Geometry: final body of the model. Coordinates: model frame, mm. A direction names the side the tool comes from. Round coordinates to 2 decimals unless told otherwise and drop trailing zeros. Loops run counter-clockwise (first coordinate to the right, second up) from the corner with the lowest first, then second, coordinate; pieces in that order, holes last. Notation, with made-up numbers: (6, 71) - (54, 71) arc R32 cw to (54, 106) - close; hole circle Ø9 at (56, -12). An arc over 180 degrees is marked (long way). Answer as CSV lines item,"result".
Autodesk Inventor part; units mm, degrees
ref_plane "YZ Plane" through (0, 0, 0) normal (1, 0, 0) x (0, 1, 0)
ref_plane "XZ Plane" through (0, 0, 0) normal (0, 1, 0) x (-1, 0, 0)
ref_plane "XY Plane" through (0, 0, 0) normal (0, 0, 1) x (1, 0, 0)
sketch "Sketch1" plane through (0, 0, 0) normal (1, 0, 0) x (0, 1, 0)
  line L0 (0, 0) -> (44.45, 0)
  line L1 (44.45, 0) -> (44.45, -6.35)
  line L2 (44.45, -6.35) -> (6.35, -6.35)
  line L3 (6.35, -6.35) -> (6.35, -19.05)
  line L4 (6.35, -19.05) -> (0, -19.05)
  line L5 (0, -19.05) -> (0, 0)
  dimension "d0" = 6.35
  dimension "d1" = 44.45
  dimension "d21" = 19.05
extrude "Extrusion1" add sketch "Sketch1" along normal blind 44.45
sketch "Sketch2" plane through (0, 0, 0) normal (0, 0, 1) x (1, 0, 0)
  line L0 (0, 44.45) -> (44.45, 44.45) construction
  line L1 (22.225, 44.45) -> (22.225, 0) construction
  line L2 (0, 0) -> (44.45, 0) construction
  point P0 (22.225, 34.925)
  dimension "d4" = 9.525
hole "Hole1" at (22.225, 34.925, 0) direction (0, 0, -1) diameter 6.7564 end through all
sketch "Sketch4" plane through (0, 6.35, -6.35) normal (0, 1, 0) x (1, 0, 0)
  line L0 (0, 6.35) -> (44.45, 6.35) construction
  line L1 (44.45, -6.35) -> (44.45, 12.7) construction
  line L2 (0, 12.7) -> (44.45, 12.7)
  line L3 (0, 0) -> (0, 12.7)
  point P0 (0, -6.35)
  point P1 (22.225, 6.35)
  point P2 (6.35, 6.35)
  point P3 (38.1, 6.35)
  dimension "d22" = 6.35
  dimension "d23" = 6.35
  dimension "d24" = 6.35
hole "Hole3" at (22.225, 6.35, -12.7) at (6.35, 6.35, -12.7) at (38.1, 6.35, -12.7) direction (0, -1, 0) diameter 5.1054 end through all
properties part number "AngleBracketForEndOfArm"
(1) Section B-B (z = -12.7). Output: boundary loops of the cut face in (x, y).
Findings below:
outline,"(0, 0) - (3.8, 0) - (3.8, 6.35) - (0, 6.35) - close; (8.9, 0) - (19.67, 0) - (19.67, 6.35) - (8.9, 6.35) - close; (24.78, 0) - (35.55, 0) - (35.55, 6.35) - (24.78, 6.35) - close; (40.65, 0) - (44.45, 0) - (44.45, 6.35) - (40.65, 6.35) - close"
(2) Access query for faces 1 (the face through (21.9, 6.35, -15.4)), 2 (the face through (22, 44.45, -3)). Directions: +Z, -Z, +X, -X, +Y, -Y. A direction counts if a zero-diameter tool reaches every point of the face in a straight line with its end or side. Return the directions, or none.
Findings below:
face 1,"-Z, +X, -X, +Y"
face 2,"+Z, -Z, +X, -X, +Y"
(3) Pin query (flat end, axial travel): P1, Ø11.5, axis at x = 19.5, y = 33, coming from the -Z side; P2, Ø1, axis at x = 15, z = -13.5, coming from the +Y side. Return the tip coordinate at first contact, or that it passes through.
Findings below:
P1,"z = -6.35"
P2,"y = 6.35"
(4) Draft query along X for faces 3 (the face through (44.45, 17, -5)), 4 (the face through (22, 22, 0)), 5 (the face through (35.57, 3.13, -13.03)). Return one class per face: pulls with the +X half, pulls with the -X half, needs draft (parallel to the pull), parting line crosses it, or undercut.
Findings below:
face 3,"pulls with the +X half"
face 4,"needs draft"
face 5,"undercut"
(5) Section A-A (x = 38.1). Output: boundary loops of the cut face in (y, z).
Findings below:
outline,"(0, -19.05) - (6.35, -19.05) - (6.35, -15.25) - (0, -15.25) - close; (0, -10.15) - (6.35, -10.15) - (6.35, -6.35) - (44.45, -6.35) - (44.45, 0) - (0, 0) - close"
(6) Section C-C (x = 23). Output: boundary loops of the cut face in (y, z), and give its area (3 significant figures).
Findings below:
outline,"(0, -19.05) - (6.35, -19.05) - (6.35, -15.13) - (0, -15.13) - close; (0, -10.27) - (6.35, -10.27) - (6.35, -6.35) - (31.64, -6.35) - (31.64, 0) - (0, 0) - close; (38.21, -6.35) - (44.45, -6.35) - (44.45, 0) - (38.21, 0) - close"
area,"290 mm2"
(7) Material intervals for line 1 along X through (y, z) = (1.75, -12.7); line 2 along Z through (x, y) = (22, 6); line 3 along Z through (x, y) = (21.5, 7.5), sorted ascending.
Findings below:
line 1,"0 to 3.8, 8.9 to 19.67, 24.78 to 35.55, 40.65 to 44.45"
line 2,"-19.05 to -15.24, -10.16 to 0"
line 3,"-6.35 to 0"
(8) Section D-D (y = 35.5). Output: boundary loops of the cut face in (x, z).
Findings below:
outline,"(0, -6.35) - (18.9, -6.35) - (18.9, 0) - (0, 0) - close; (25.55, -6.35) - (44.45, -6.35) - (44.45, 0) - (25.55, 0) - close"
